Design review of the part built by this model. Coordinates are the model's own, in mm. Face numbers are marked on the shaded views. Round coordinates to 2 decimals unless told otherwise and drop trailing zeros. Order: outer loops, then holes, each group sorted by start corner. A loop starts at its lowest first (then second) coordinate and runs counter-clockwise, first axis right, second up. Notation, with made-up numbers: M 56,-34 L 87,-34 A22 ccw 87,-3 Z; hole C -29.5,62 d9. An arc over 180 degrees is marked long. Use a Markdown table: item, result. Add a question column.
(1) Take a section at C-C (x = 35). Write out the cut boundary in (y, z), then the cut area to 3 significant figures.
(2) For pin 1 (2 mm diameter, centred on x = 19, y = -6.5, fed in from +Z); pin 2 (3 mm diameter, centred on x = -34.5, z = 3.5, fed in from +Y); pin 3 (2 mm diameter, centred on x = 51.5, z = 4.5, fed in from -Y), all flat-tipped, find the tip position at first contact; note any pin that passes through.
(3) Take a section at D-D (y = 46.25). Write out the cut boundary in (x, z), then the cut area to 3 significant figures.
(4) Take a section at A-A (y = 0). Write out the cut boundary in (x, z) (3 decimals).
(5) The part is to be moulded in two halves that separate along Y. For the marked faces 1 and 2, say which applies: released by +Y, released by -Y, zero draft, split by the parting line, or undercut.
(6) To check wall thickness, follow probe 1 along Y at (x, z) = (0, -0.7); probe 2 along Y at (x, z) = (0, 2.25) (3 decimals); probe 3 along Y at (x, z) = (0, 4.35) (3 decimals). State the ranges of each line that lie inside material, in increasing order. Write a range as from..to.
(7) Take a section at B-B (x = 0). Count the separate pieces of the cut face and the enclosed holes in it, then the cut area to 3 significant figures.
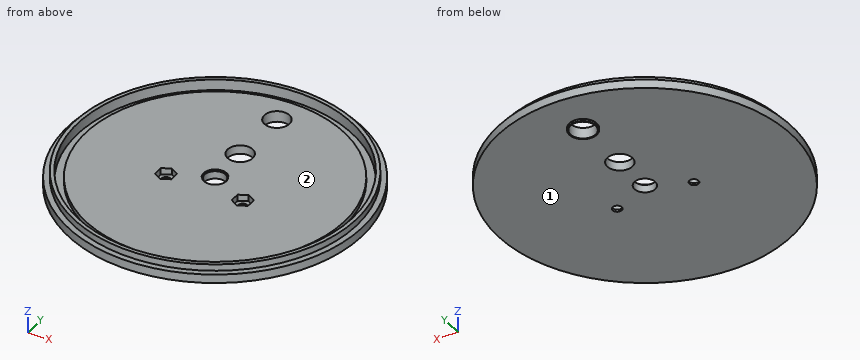
```python
from build123d import *

# Parameters (mm, degrees)
F0_R      = 67
F1_DEPTH  = 2.5
F2_R      = 64.375
F2_R_2    = 62.625
F3_DEPTH  = 3
F2_R_3    = 58.875
F4_DEPTH  = 2
F5_R      = 4.75
F5_R_2    = 5.75
F5_R_3    = 2.1
F6_DEPTH  = 5.001
F7_R      = 5.25
F7_R_2    = 4.75
F8_DEPTH  = 0.5
F7_R_3    = 2.1
F9_DEPTH  = 3
F10_DEPTH = 3
F11_R     = 67
F11_R_2   = 6.25
F11_R_3   = 2.1
F11_R_4   = 4.75
F11_R_5   = 5.75
F12_DEPTH = 1


with BuildPart() as f1:
    # F0 (on Top) → F1 (new body, symmetric)
    with BuildSketch(Plane.XY):
        Circle(F0_R)
    extrude(amount=F1_DEPTH, both=True)

    # F2 (on face) → F3 (join)
    with BuildSketch(Plane.XY.offset(2.5)):
        Circle(F2_R)
        Circle(F2_R_2, mode=Mode.SUBTRACT)
    extrude(amount=F3_DEPTH)

    # F2 (on face) → F4 (cut)
    with BuildSketch(Plane.XY.offset(2.5)):
        Circle(F2_R_2)
        Circle(F2_R_3, mode=Mode.SUBTRACT)
    extrude(amount=-F4_DEPTH, mode=Mode.SUBTRACT)

    # F5 (on face) → F6 (cut, through all)
    with BuildSketch(Plane.XY.offset(2.5)):
        Circle(F5_R)
        with Locations((0, 18.75)):
            Circle(F5_R_2)
        with Locations((0, 46.25)):
            Circle(F5_R_2)
        with Locations((17.5, -8)):
            Circle(F5_R_3)
        with Locations((-17.5, -8)):
            Circle(F5_R_3)
    extrude(amount=-F6_DEPTH, mode=Mode.SUBTRACT)

    # F7 (on face) → F8 (cut)
    with BuildSketch(Plane.XY.offset(2.5)):
        Circle(F7_R)
        Circle(F7_R_2, mode=Mode.SUBTRACT)
    extrude(amount=-F8_DEPTH, mode=Mode.SUBTRACT)

    # F7 (on face) → F9 (cut)
    with BuildSketch(Plane.XY.offset(2.5)):
        Polygon((-13.75, -10.1650635095), (-13.75, -5.8349364905), (-17.5, -3.6698729811), (-21.25, -5.8349364905), (-21.25, -10.1650635095), (-17.5, -12.3301270189), align=None)
        with Locations((-17.5, -8)):
            Circle(F7_R_3, mode=Mode.SUBTRACT)
        with Locations((-17.5, -8)):
            Circle(F7_R_3)
    extrude(amount=-F9_DEPTH, mode=Mode.SUBTRACT)

    # F7 (on face) → F10 (cut)
    with BuildSketch(Plane.XY.offset(2.5)):
        Polygon((17.5, -12.3301270189), (21.25, -10.1650635095), (21.25, -5.8349364905), (17.5, -3.6698729811), (13.75, -5.8349364905), (13.75, -10.1650635095), align=None)
        with Locations((17.5, -8)):
            Circle(F7_R_3, mode=Mode.SUBTRACT)
        with Locations((17.5, -8)):
            Circle(F7_R_3)
    extrude(amount=-F10_DEPTH, mode=Mode.SUBTRACT)

    # F11 (on face) → F12 (cut)
    with BuildSketch(Plane(origin=(0, 0, -2.5), x_dir=(1, 0, 0), z_dir=(0, 0, -1))):
        Circle(F11_R)
        with Locations((0, -46.25)):
            Circle(F11_R_2, mode=Mode.SUBTRACT)
        with Locations((0, -18.75)):
            Circle(F11_R_2, mode=Mode.SUBTRACT)
        with Locations((-17.5, 8)):
            Circle(F11_R_3, mode=Mode.SUBTRACT)
        Circle(F11_R_4, mode=Mode.SUBTRACT)
        with Locations((17.5, 8)):
            Circle(F11_R_3, mode=Mode.SUBTRACT)
        with Locations((0, -18.75)):
            Circle(F11_R_2)
        with Locations((0, -18.75)):
            Circle(F11_R_5, mode=Mode.SUBTRACT)
    extrude(amount=-F12_DEPTH, mode=Mode.SUBTRACT)


solid = f1.part
```
Verdict:
| question | item | result |
|---|---|---|
| 1 | outline | M -57.13,-1.5 L 57.13,-1.5 L 57.13,2.5 L 54.03,2.5 L 54.03,5.5 L 51.93,5.5 L 51.93,0.5 L 47.34,0.5 L 47.34,2.5 L -47.34,2.5 L -47.34,0.5 L -51.93,0.5 L -51.93,5.5 L -54.03,5.5 L -54.03,2.5 L -57.13,2.5 Z |
| 1 | area | 451 mm^2 |
| 2 | pin 1 | stops at z = -0.5 |
| 2 | pin 2 | stops at y = 58.09 |
| 2 | pin 3 | stops at y = -39.92 |
| 3 | outline | M -48.48,-1.5 L -6.25,-1.5 L -6.25,-2.5 L -5.75,-2.5 L -5.75,2.5 L -36.43,2.5 L -36.43,0.5 L -42.22,0.5 L -42.22,5.5 L -44.78,5.5 L -44.78,2.5 L -48.48,2.5 Z; M 5.75,-2.5 L 6.25,-2.5 L 6.25,-1.5 L 48.48,-1.5 L 48.48,2.5 L 44.78,2.5 L 44.78,5.5 L 42.22,5.5 L 42.22,0.5 L 36.43,0.5 L 36.43,2.5 L 5.75,2.5 Z |
| 3 | area | 335 mm^2 |
| 4 | outline | M -67,-1.5 L -4.75,-1.5 L -4.75,2 L -5.25,2 L -5.25,2.5 L -58.875,2.5 L -58.875,0.5 L -62.625,0.5 L -62.625,5.5 L -64.375,5.5 L -64.375,2.5 L -67,2.5 Z; M 4.75,-1.5 L 67,-1.5 L 67,2.5 L 64.375,2.5 L 64.375,5.5 L 62.625,5.5 L 62.625,0.5 L 58.875,0.5 L 58.875,2.5 L 5.25,2.5 L 5.25,2 L 4.75,2 Z |
| 5 | face 1 | zero draft |
| 5 | face 2 | undercut |
| 6 | probe 1 | y = -67..-4.75, 4.75..13, 24.5..40.5, 52..67 |
| 6 | probe 2 | y = -67..-62.625, -58.875..-5.25, 5.25..13, 24.5..40.5, 52..58.875, 62.625..67 |
| 6 | probe 3 | y = -64.375..-62.625, 62.625..64.375 |
| 7 | separate pieces | 4 |
| 7 | enclosed holes | 0 |
| 7 | area | 402 mm^2 |
